Input: part model. Units: mm. Frame: model coordinates. Give positions to 0.01 mm unless a question says otherwise; leave off trailing zeros. Loops run counter-clockwise (first coordinate to the right, second up) from the corner with the lowest first, then second, coordinate; pieces in that order, holes last. Notation, with made-up numbers: M 36.5,77.25 L 69.5,77.25 A13 ccw 69.5,97.25 Z; hole C 12.5,-36.5 d8. An arc over 180 degrees is marked long. One line per item, written item: value. Start each with the question number.
(1) Pull-direction query (Y, two-part tool) for faces 1 (the flat face through (-99, 76.5, 3)), 2 (the cylindrical face through (-187.474, 65.352, 3.042)), 3 (the cylindrical face through (-197.15, -13.49, 3.04)); classes: released by +Y, released by -Y, zero draft, split by the parting line, or undercut.
(2) Section B-B on z = 3.65. State how many separate pieces and enclosed holes the cut face has, plus the area to 3 significant figures.
(3) Section A-A on x = -186. Output: boundary loops of the cut face in (y, z), plus the area to 3 significant figures.
(4) Ray query, line 1 along Y through (x, z) = (-114.4, 1.45); line 2 along Y through (x, z) = (-97.9, 4); line 3 along X through (y, z) = (-7, 1.05). Return the intervals inside material, ascending. Write a range as from..to.
(5) Pin query (flat end, axial travel): P1, Ø2.5, axis at x = -14, y = -4, coming from the +Z side. Return the tip coordinate at first contact, or that it passes through.
```python
from build123d import *

# Parameters (mm, degrees)
EXTRUDE_1_DEPTH     = 6
SKETCH_10_R         = 1.5
CUT_EXTRUDE_1_DEPTH = 6
CUT_EXTRUDE_2_REACH = 216.215
SKETCH_11_R         = 2
FILLET_1_R          = 10


with BuildPart() as part:
    # 草圖1 → 填料-伸長1 (new body)
    with BuildSketch(Plane.XY):
        Polygon((-200, 60), (-200, 76.5), (-168.2, 76.5), (-125.9, 76.5), (-94.1, 76.5), (-51.8, 76.5), (0, 76.5), (0, 60), (0, 0), (0, -16.5), (-51.8, -16.5), (-94.1, -16.5), (-125.9, -16.5), (-168.2, -16.5), (-200, -16.5), (-200, 0), align=None)
    extrude(amount=EXTRUDE_1_DEPTH)

    # 草圖10 → 除料-伸長1 (cut)
    with BuildSketch(Plane.XY.offset(6)):
        with Locations((-164.75, 54.3)):
            Circle(SKETCH_10_R)
        with Locations((-123.85, 39.25)):
            Circle(SKETCH_10_R)
        with Locations((-123.85, 10.975)):
            Circle(SKETCH_10_R)
        with Locations((-97.9, 50)):
            Circle(SKETCH_10_R)
        with Locations((-66.45, 50)):
            Circle(SKETCH_10_R)
        with Locations((-51.45, 50)):
            Circle(SKETCH_10_R)
        with Locations((-20, 50)):
            Circle(SKETCH_10_R)
        with Locations((-20, 10)):
            Circle(SKETCH_10_R)
        with Locations((-51.45, 10)):
            Circle(SKETCH_10_R)
        with Locations((-66.45, 10)):
            Circle(SKETCH_10_R)
        with Locations((-97.9, 10)):
            Circle(SKETCH_10_R)
    extrude(amount=-CUT_EXTRUDE_1_DEPTH, mode=Mode.SUBTRACT)

    # 草圖11 → 除料-伸長2 (cut, up to next)
    with BuildSketch(Plane.XY.offset(6), mode=Mode.PRIVATE) as cut_extrude_2_sk1:
        with Locations((-14, 64)):
            Circle(SKETCH_11_R)
    cut_extrude_2_tool1 = extrude(cut_extrude_2_sk1.sketch, amount=-CUT_EXTRUDE_2_REACH, mode=Mode.PRIVATE) & part.part
    # 草圖11 → 除料-伸長2 (cut, up to next)
    with BuildSketch(Plane.XY.offset(6), mode=Mode.PRIVATE) as cut_extrude_2_sk2:
        with Locations((-42.8, 64)):
            Circle(SKETCH_11_R)
    cut_extrude_2_tool2 = extrude(cut_extrude_2_sk2.sketch, amount=-CUT_EXTRUDE_2_REACH, mode=Mode.PRIVATE) & part.part
    # 草圖11 → 除料-伸長2 (cut, up to next)
    with BuildSketch(Plane.XY.offset(6), mode=Mode.PRIVATE) as cut_extrude_2_sk3:
        with Locations((-85.6, 64)):
            Circle(SKETCH_11_R)
    cut_extrude_2_tool3 = extrude(cut_extrude_2_sk3.sketch, amount=-CUT_EXTRUDE_2_REACH, mode=Mode.PRIVATE) & part.part
    # 草圖11 → 除料-伸長2 (cut, up to next)
    with BuildSketch(Plane.XY.offset(6), mode=Mode.PRIVATE) as cut_extrude_2_sk4:
        with Locations((-114.4, 64)):
            Circle(SKETCH_11_R)
    cut_extrude_2_tool4 = extrude(cut_extrude_2_sk4.sketch, amount=-CUT_EXTRUDE_2_REACH, mode=Mode.PRIVATE) & part.part
    # 草圖11 → 除料-伸長2 (cut, up to next)
    with BuildSketch(Plane.XY.offset(6), mode=Mode.PRIVATE) as cut_extrude_2_sk5:
        with Locations((-157.2, 64)):
            Circle(SKETCH_11_R)
    cut_extrude_2_tool5 = extrude(cut_extrude_2_sk5.sketch, amount=-CUT_EXTRUDE_2_REACH, mode=Mode.PRIVATE) & part.part
    # 草圖11 → 除料-伸長2 (cut, up to next)
    with BuildSketch(Plane.XY.offset(6), mode=Mode.PRIVATE) as cut_extrude_2_sk6:
        with Locations((-186, 64)):
            Circle(SKETCH_11_R)
    cut_extrude_2_tool6 = extrude(cut_extrude_2_sk6.sketch, amount=-CUT_EXTRUDE_2_REACH, mode=Mode.PRIVATE) & part.part
    # 草圖11 → 除料-伸長2 (cut, up to next)
    with BuildSketch(Plane.XY.offset(6), mode=Mode.PRIVATE) as cut_extrude_2_sk7:
        with Locations((-14, -4)):
            Circle(SKETCH_11_R)
    cut_extrude_2_tool7 = extrude(cut_extrude_2_sk7.sketch, amount=-CUT_EXTRUDE_2_REACH, mode=Mode.PRIVATE) & part.part
    # 草圖11 → 除料-伸長2 (cut, up to next)
    with BuildSketch(Plane.XY.offset(6), mode=Mode.PRIVATE) as cut_extrude_2_sk8:
        with Locations((-42.8, -4)):
            Circle(SKETCH_11_R)
    cut_extrude_2_tool8 = extrude(cut_extrude_2_sk8.sketch, amount=-CUT_EXTRUDE_2_REACH, mode=Mode.PRIVATE) & part.part
    # 草圖11 → 除料-伸長2 (cut, up to next)
    with BuildSketch(Plane.XY.offset(6), mode=Mode.PRIVATE) as cut_extrude_2_sk9:
        with Locations((-85.6, -4)):
            Circle(SKETCH_11_R)
    cut_extrude_2_tool9 = extrude(cut_extrude_2_sk9.sketch, amount=-CUT_EXTRUDE_2_REACH, mode=Mode.PRIVATE) & part.part
    # 草圖11 → 除料-伸長2 (cut, up to next)
    with BuildSketch(Plane.XY.offset(6), mode=Mode.PRIVATE) as cut_extrude_2_sk10:
        with Locations((-114.4, -4)):
            Circle(SKETCH_11_R)
    cut_extrude_2_tool10 = extrude(cut_extrude_2_sk10.sketch, amount=-CUT_EXTRUDE_2_REACH, mode=Mode.PRIVATE) & part.part
    # 草圖11 → 除料-伸長2 (cut, up to next)
    with BuildSketch(Plane.XY.offset(6), mode=Mode.PRIVATE) as cut_extrude_2_sk11:
        with Locations((-157.2, -4)):
            Circle(SKETCH_11_R)
    cut_extrude_2_tool11 = extrude(cut_extrude_2_sk11.sketch, amount=-CUT_EXTRUDE_2_REACH, mode=Mode.PRIVATE) & part.part
    # 草圖11 → 除料-伸長2 (cut, up to next)
    with BuildSketch(Plane.XY.offset(6), mode=Mode.PRIVATE) as cut_extrude_2_sk12:
        with Locations((-186, -4)):
            Circle(SKETCH_11_R)
    cut_extrude_2_tool12 = extrude(cut_extrude_2_sk12.sketch, amount=-CUT_EXTRUDE_2_REACH, mode=Mode.PRIVATE) & part.part
    add(cut_extrude_2_tool1.solids().sort_by_distance((-14, 64, 6))[0], mode=Mode.SUBTRACT)
    add(cut_extrude_2_tool2.solids().sort_by_distance((-42.8, 64, 6))[0], mode=Mode.SUBTRACT)
    add(cut_extrude_2_tool3.solids().sort_by_distance((-85.6, 64, 6))[0], mode=Mode.SUBTRACT)
    add(cut_extrude_2_tool4.solids().sort_by_distance((-114.4, 64, 6))[0], mode=Mode.SUBTRACT)
    add(cut_extrude_2_tool5.solids().sort_by_distance((-157.2, 64, 6))[0], mode=Mode.SUBTRACT)
    add(cut_extrude_2_tool6.solids().sort_by_distance((-186, 64, 6))[0], mode=Mode.SUBTRACT)
    add(cut_extrude_2_tool7.solids().sort_by_distance((-14, -4, 6))[0], mode=Mode.SUBTRACT)
    add(cut_extrude_2_tool8.solids().sort_by_distance((-42.8, -4, 6))[0], mode=Mode.SUBTRACT)
    add(cut_extrude_2_tool9.solids().sort_by_distance((-85.6, -4, 6))[0], mode=Mode.SUBTRACT)
    add(cut_extrude_2_tool10.solids().sort_by_distance((-114.4, -4, 6))[0], mode=Mode.SUBTRACT)
    add(cut_extrude_2_tool11.solids().sort_by_distance((-157.2, -4, 6))[0], mode=Mode.SUBTRACT)
    add(cut_extrude_2_tool12.solids().sort_by_distance((-186, -4, 6))[0], mode=Mode.SUBTRACT)

    # 圓角1
    fillet_1_edges = [part.edges().sort_by_distance(p)[0] for p in [
        (0, -16.5, 3),
        (-200, -16.5, 3),
        (-200, 76.5, 3),
        (0, 76.5, 3),
    ]]
    fillet(fillet_1_edges, radius=FILLET_1_R)


solid = part.part
```
Output values:
1. face 1: released by +Y
1. face 2: undercut
1. face 3: released by -Y
2. separate pieces: 1
2. enclosed holes: 23
2. area: 18,300 mm²
3. outline: M -16.5,0 L -6,0 L -6,6 L -16.5,6 Z; M -2,0 L 62,0 L 62,6 L -2,6 Z; M 66,0 L 76.5,0 L 76.5,6 L 66,6 Z
3. area: 510 mm²
4. line 1: y = -16.5..-6, -2..62, 66..76.5
4. line 2: y = -16.5..8.5, 11.5..48.5, 51.5..76.5
4. line 3: x = -199.99..-0.01
5. P1: passes through
